```python
from build123d import *

# Parameters (mm, degrees)
F0_W     = 26
F0_H     = 2
F1_DEPTH = 40
F2_R     = 0.99999
F3_R     = 12.99999
F4_R     = 15


# Not quite as in the source:
# - a fillet or chamfer is up to 0.001 mm smaller than in the source, because OpenCascade refuses the exact size


with BuildPart() as f1:
    # F0 (on Top) → F1 (new body)
    with BuildSketch(Plane.XY):
        Polygon((-24.5838956386, 17.7643506003), (-26.5838956386, 17.7643506003), (-26.5838956386, -12.2356493997), (-24.5838956386, -12.2356493997), (-24.5838956386, -10.2356493997), align=None)
        with Locations((-11.5838956386, -11.2356493997)):
            Rectangle(F0_W, F0_H)
        Polygon((1.4161043614, 37.7643506003), (1.4161043614, -10.2356493997), (1.4161043614, -12.2356493997), (3.4161043614, -12.2356493997), (3.4161043614, 37.7643506003), align=None)
    extrude(amount=F1_DEPTH)

    # F2 (radius 1 in the source; OpenCascade refuses exactly that, so slightly less here)
    f2_edges = [f1.edges().sort_by_distance(p)[0] for p in [
        (-26.583896, 17.764351, 20),
        (-24.583896, 17.764351, 20),
        (1.416104, 37.764351, 20),
    ]]
    fillet(f2_edges, radius=F2_R)

    # F3 (radius 13 in the source; OpenCascade refuses exactly that, so slightly less here)
    f3_edges = [f1.edges().sort_by_distance(p)[0] for p in [
        (1.416104, -10.235649, 20),
        (-24.583896, -10.235649, 20),
    ]]
    fillet(f3_edges, radius=F3_R)

    # F4
    f4_edges = [f1.edges().sort_by_distance(p)[0] for p in [
        (-26.583896, -12.235649, 20),
    ]]
    fillet(f4_edges, radius=F4_R)


solid = f1.part
```
The listing builds one solid part. Answer for the finished solid, in the listing's coordinates (mm). A direction names the side the tool comes from. Give positions to 0.01 mm unless a question says otherwise; leave off trailing zeros. Order: outer loops, then holes, each group sorted by start corner. A loop starts at its lowest first (then second) coordinate and runs counter-clockwise, first axis right, second up. Notation, with made-up numbers: (70.25, 56.5) - (125.25, 56.5) arc R31 ccw to (125.25, 81.5) - close; hole circle Ø8 at (53, -1). An arc over 180 degrees is marked (long way). Answer in a Markdown table with one row per item. Add a question column.
Q1. Given P1, Ø8, axis at x = -7, z = 22.5, coming from the +Y side; P2, Ø10, axis at x = -13.5, z = 34.5, coming from the +Y side; P3, Ø4, axis at x = -4, z = 21.5, coming from the +Y side, each flat-ended and moving along its own axis, determine where each tip first touches the part or whether it passes through.
Q2. The part is cut by section A-A (y = 14.5). Determine the outline of the cut face in (x, z).
Q3. Find the intervals of material crossed by line 1 along X through (y, z) = (14.5, 9.5); line 2 along X through (y, z) = (24, 37); line 3 along X through (y, z) = (-7.5, 26), in increasing order. Write a range as [from, to].
Q4. The part is cut by section C-C (y = 0). Determine the outline of the cut face in (x, z).
Q5. Which of the six approach directions +Z, -Z, +X, -X, +Y, -Y give full straight-line access (tool end or side, diameter ignored) to faces 4 (the cylindrical face through (-22.31, -7.72, 20.28)), 5 (the flat face through (-24.584, 10, 20))?
Q6. The part is cut by section D-D (x = -8). Determine the outline of the cut face in (y, z), then the cut area to 3 significant figures.
Q7. For a pull along X with two mould halves and no side action, classify faces 1 (the flat face through (3.416, 12, 20)), 2 (the flat face through (1.416, 20, 20)), 3 (the flat face through (-26.584, 10, 20)) as released by +X, released by -X, zero draft, split by the parting line, or undercut.
Determined:
| question | item | result |
|---|---|---|
| 1 | P1 | stops at y = -7 |
| 1 | P2 | stops at y = -8.24 |
| 1 | P3 | stops at y = -6.02 |
| 2 | outline | (-26.58, 0) - (-24.58, 0) - (-24.58, 40) - (-26.58, 40) - close; (1.42, 0) - (3.42, 0) - (3.42, 40) - (1.42, 40) - close |
| 3 | line 1 | x = [-26.58, -24.58], [1.42, 3.42] |
| 3 | line 2 | x = [1.42, 3.42] |
| 3 | line 3 | x = [-22.52, -19.56], [-3.61, 3.42] |
| 4 | outline | (-26.33, 0) - (-24.29, 0) - (-24.29, 40) - (-26.33, 40) - close; (1.12, 0) - (3.42, 0) - (3.42, 40) - (1.12, 40) - close |
| 5 | face 4 | +Z, -Z, -X, -Y |
| 5 | face 5 | +Z, -Z, +Y |
| 6 | outline | (-12.24, 0) - (-9.73, 0) - (-9.73, 40) - (-12.24, 40) - close |
| 6 | area | 100 mm² |
| 7 | face 1 | released by +X |
| 7 | face 2 | undercut |
| 7 | face 3 | released by -X |
